from build123d import *

# Parameters (mm, degrees)
SKETCH1_W           = 145
SKETCH1_H           = 21
BOSS_EXTRUDE1_DEPTH = 3
SKETCH2_W           = 12
SKETCH2_H           = 11
CUT_EXTRUDE1_DEPTH  = 147.543508898
SKETCH3_R           = 2.25
CUT_EXTRUDE2_DEPTH  = 147.543508898
SKETCH4_R           = 0.5
CUT_EXTRUDE3_DEPTH  = 147.543508898
SKETCH5_W           = 10
SKETCH5_H           = 3
BOSS_EXTRUDE2_DEPTH = 3
LPATTERN1_COUNT     = 4
LPATTERN1_PITCH     = 20
LPATTERN1_COL_COUNT = 4
LPATTERN1_COL_PITCH = 20
SKETCH6_W           = 145
SKETCH6_H           = 3
BOSS_EXTRUDE3_DEPTH = 3
SKETCH8_W           = 10
SKETCH8_H           = 3
CUT_EXTRUDE4_DEPTH  = 148.522879581
SKETCH9_W           = 3
SKETCH9_H           = 5
CUT_EXTRUDE5_DEPTH  = 148.522879581
SKETCH10_W          = 13
SKETCH10_H          = 3
CUT_EXTRUDE6_DEPTH  = 148.522879581


with BuildPart() as part:
    # Sketch1 → Boss-Extrude1 (new body)
    with BuildSketch(Plane(origin=(0, 0, 0), x_dir=(1, 0, 0), z_dir=(0, 1, 0))):
        with Locations((72.5, -10.5)):
            Rectangle(SKETCH1_W, SKETCH1_H)
    extrude(amount=BOSS_EXTRUDE1_DEPTH)

    # Sketch2 → Cut-Extrude1 (cut, through all)
    with BuildSketch(Plane(origin=(0, 3, 0), x_dir=(1, 0, 0), z_dir=(0, 1, 0))):
        with Locations((72.5, -10)):
            Rectangle(SKETCH2_W, SKETCH2_H)
    extrude(amount=-CUT_EXTRUDE1_DEPTH, mode=Mode.SUBTRACT)

    # Sketch3 → Cut-Extrude2 (cut, through all)
    with BuildSketch(Plane(origin=(0, 3, 0), x_dir=(1, 0, 0), z_dir=(0, 1, 0))):
        with Locations(Location((42, -4, 0), (0, 0, 270))):
            Circle(SKETCH3_R)
        with Locations(Location((130, -4, 0), (0, 0, 270))):
            Circle(SKETCH3_R)
    extrude(amount=-CUT_EXTRUDE2_DEPTH, mode=Mode.SUBTRACT)

    # Sketch4 → Cut-Extrude3 (cut, through all)
    with BuildSketch(Plane(origin=(0, 3, 0), x_dir=(1, 0, 0), z_dir=(0, 1, 0))):
        with BuildLine():
            Line((98.5, -7), (98.5, -16))
            Line((98.5, -16), (105.5, -16))
            ThreePointArc((105.5, -16), (110, -11.500000006), (105.500000011, -7))
            Line((105.500000011, -7), (98.5, -7))
        make_face()
        with Locations(Location((96.75, -11.5, 0), (0, 0, 270))):
            Circle(SKETCH4_R)
        with Locations(Location((111.75, -11.5, 0), (0, 0, 270))):
            Circle(SKETCH4_R)
    extrude(amount=-CUT_EXTRUDE3_DEPTH, mode=Mode.SUBTRACT)

    # Sketch5 → Boss-Extrude2 (add, through all)
    with BuildSketch(Plane(origin=(0, 3, 0), x_dir=(1, 0, 0), z_dir=(0, 1, 0))):
        with Locations((72.5, -22.5)):
            Rectangle(SKETCH5_W, SKETCH5_H)
        with Locations((72.5, 1.5)):
            Rectangle(SKETCH5_W, SKETCH5_H)
    boss_extrude2 = extrude(amount=-BOSS_EXTRUDE2_DEPTH)

    # LPattern1: Boss-Extrude2 ×4
    with Locations(*[(-i * LPATTERN1_PITCH, 0, 0) for i in range(1, LPATTERN1_COUNT)]):
        add(boss_extrude2)

    # LPattern1 col: Boss-Extrude2 ×4
    with Locations(*[(i * LPATTERN1_COL_PITCH, 0, 0) for i in range(1, LPATTERN1_COL_COUNT)]):
        add(boss_extrude2)

    # Sketch6 → Boss-Extrude3 (add, through all)
    with BuildSketch(Plane(origin=(0, 3, 0), x_dir=(1, 0, 0), z_dir=(0, 1, 0))):
        with Locations((72.5, -25.5)):
            Rectangle(SKETCH6_W, SKETCH6_H)
    extrude(amount=-BOSS_EXTRUDE3_DEPTH)

    # Sketch8 → Cut-Extrude4 (cut, through all)
    with BuildSketch(Plane(origin=(0, 0, 0), x_dir=(-1, 0, 0), z_dir=(0, -1, 0))):
        with Locations((-12.5, -22.5)):
            Rectangle(SKETCH8_W, SKETCH8_H)
        with Locations((-132.5, -22.5)):
            Rectangle(SKETCH8_W, SKETCH8_H)
    extrude(amount=-CUT_EXTRUDE4_DEPTH, mode=Mode.SUBTRACT)

    # Sketch9 → Cut-Extrude5 (cut, through all)
    with BuildSketch(Plane(origin=(0, 3, 0), x_dir=(1, 0, 0), z_dir=(0, 1, 0))):
        with Locations((1.5, -15.5)):
            Rectangle(SKETCH9_W, SKETCH9_H)
        with Locations((1.5, -5.5)):
            Rectangle(SKETCH9_W, SKETCH9_H)
        with Locations((143.5, -15.5)):
            Rectangle(SKETCH9_W, SKETCH9_H)
        with Locations((143.5, -5.5)):
            Rectangle(SKETCH9_W, SKETCH9_H)
    extrude(amount=-CUT_EXTRUDE5_DEPTH, mode=Mode.SUBTRACT)

    # Sketch10 → Cut-Extrude6 (cut, through all)
    with BuildSketch(Plane(origin=(0, 0, 0), x_dir=(-1, 0, 0), z_dir=(0, -1, 0))):
        with Locations((-6.5, -25.5)):
            Rectangle(SKETCH10_W, SKETCH10_H)
        with Locations((-138.5, -25.5)):
            Rectangle(SKETCH10_W, SKETCH10_H)
    extrude(amount=-CUT_EXTRUDE6_DEPTH, mode=Mode.SUBTRACT)


solid = part.part
Input: part model. Units: mm. Frame: model coordinates. A direction names the side the tool comes from. Coordinates: 2 decimals unless noted, no trailing zeros. Loops run counter-clockwise (first coordinate to the right, second up) from the corner with the lowest first, then second, coordinate; pieces in that order, holes last.
(1) First-contact query: pin 1 Ø0.9 at (x, y) = (143.5, 1.5) entering from +Z; pin 2 Ø1.5 at (y, z) = (1.5, -1.5) entering from -X; pin 3 Ø1.5 at (y, z) = (1.5, 23) entering from -X. Flat tips, straight axial feed; report the tip coordinate or a pass-through.
(2) Pull-direction query (X, two-part tool) for faces 4 (the face through (0, 1, 20)), 5 (the face through (97.5, 2, 23)), 6 (the face through (131, 1, 21)); classes: released by +X, released by -X, zero draft, split by the parting line, or undercut.
(3) Section A-A on x = 130. Return the cut outline in (y, z), then the cut area to 3 significant figures.
(4) Section C-C on x = 20. Return the cut outline in (y, z).
(5) Material intervals for probe 1 along X at (y, z) = (0.9, 4); probe 2 along Z at (x, y) = (130, 1.65); probe 3 along X at (y, z) = (2.35, 11.5), sorted ascending.
(6) Set-up query: faces 1 (the face through (117.5, 2, 23)), 2 (the face through (78.5, 2, 10)), 3 (the face through (42, 1, 0)). Return all of +Z, -Z, +X, -X, +Y, -Y with unobstructed straight access to the full face (end or side cutting, diameter ignored); none if empty.
(7) Section B-B on z = 22.75. Return the cut outline in (x, y).
(8) Section D-D on x = 101. Return the cut outline in (y, z), then the cut area to 3 significant figures.
Data:
1. pin 1: stops at z = 21
1. pin 2: stops at x = 7.5
1. pin 3: stops at x = 27.5
2. face 4: released by -X
2. face 5: undercut
2. face 6: zero draft
3. outline: (0, -3) - (3, -3) - (3, 1.75) - (0, 1.75) - close; (0, 6.25) - (3, 6.25) - (3, 21) - (0, 21) - close; (0, 24) - (3, 24) - (3, 27) - (0, 27) - close
3. area: 67.5 mm2
4. outline: (0, 0) - (3, 0) - (3, 21) - (0, 21) - close; (0, 24) - (3, 24) - (3, 27) - (0, 27) - close
5. probe 1: x = 3 to 39.75, 44.25 to 127.75, 132.25 to 142
5. probe 2: z = -3 to 1.75, 6.25 to 21, 24 to 27
5. probe 3: x = 0 to 66.5, 78.5 to 96.25, 97.25 to 98.5, 110 to 111.25, 112.25 to 145
6. face 1: +X, +Y, -Y
6. face 2: +Y, -Y
6. face 3: -Z, +Y, -Y
7. outline: (27.5, 0) - (37.5, 0) - (37.5, 3) - (27.5, 3) - close; (47.5, 0) - (57.5, 0) - (57.5, 3) - (47.5, 3) - close; (67.5, 0) - (77.5, 0) - (77.5, 3) - (67.5, 3) - close; (87.5, 0) - (97.5, 0) - (97.5, 3) - (87.5, 3) - close; (107.5, 0) - (117.5, 0) - (117.5, 3) - (107.5, 3) - close
8. outline: (0, 0) - (3, 0) - (3, 7) - (0, 7) - close; (0, 16) - (3, 16) - (3, 21) - (0, 21) - close; (0, 24) - (3, 24) - (3, 27) - (0, 27) - close
8. area: 45.0 mm2
